Part print with two shaded views. Sizes in mm from the minimum x, y, z corner. A direction names the side the tool comes from. Round coordinates to 2 decimals unless told otherwise and drop trailing zeros. Write each loop counter-clockwise with the first axis right and the second up, starting at its lowest first coordinate (ties: lowest second). Pieces come first, ordered by that corner, then holes.
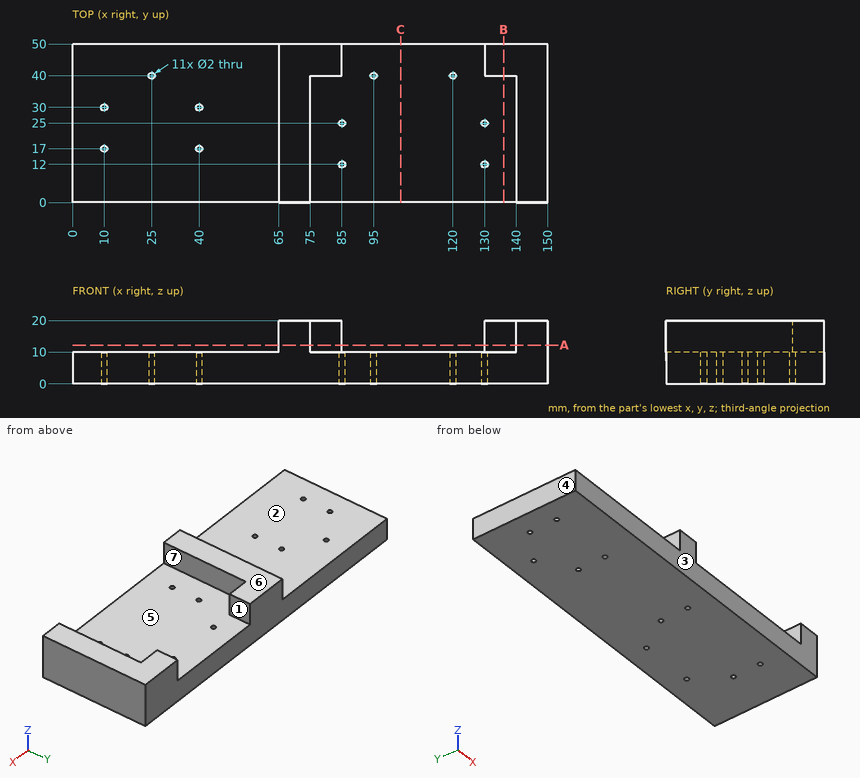
Q1. Wall check: L1, parallel to X at y = 12, z = 5.5; L2, parallel to Y at x = 130, z = 4.25; L3, parallel to Y at x = 10, z = 5.5. Give the ranges that are in metal, low to high.
Values follow:
L1: x = 0 to 84, 86 to 129, 131 to 150
L2: y = 0 to 11, 13 to 24, 26 to 50
L3: y = 0 to 16, 18 to 29, 31 to 50
Q2. Cut at A-A on z = 12.25. Write the cut outline in (x, y), plus the area to 3 significant figures.
Values follow:
outline: (65, 0) - (75, 0) - (75, 40) - (85, 40) - (85, 50) - (65, 50) - close; (130, 40) - (140, 40) - (140, 0) - (150, 0) - (150, 50) - (130, 50) - close
area: 1,200 mm2
Q3. Drop flat-ended pins along their axis: pin 1 (2.5 mm diameter, centred on x = 10, y = 30, fed in from +Z); pin 2 (3 mm diameter, centred on y = 16.5, z = 13.5, fed in from -X). Give the stop position or say it passes through.
Values follow:
pin 1: stops at z = 10
pin 2: stops at x = 65
Q4. Mould opens along X. For the marked faces 4, 5, 6 and 7 say: +X half, -X half, draft (parallel to the pull), parting line (faces both ways), or undercut.
Values follow:
face 4: -X half
face 5: undercut
face 6: draft
face 7: undercut
Q5. Cut at C-C on x = 103.5. Write the cut outline in (y, z), plus the area to 3 significant figures.
Values follow:
outline: (0, 0) - (50, 0) - (50, 10) - (0, 10) - close
area: 500 mm2
Q6. Which spindle directions (+Z, -Z, +X, -X, +Y, -Y) get a long thin tool onto all of the face, cutting with end or side? Do the marked faces 1, 2 and 3. Say none if no direction does.
Values follow:
face 1: +Z, +Y, -Y
face 2: +Z, -X, +Y, -Y
face 3: +Z, -Z, +X, -X, -Y
Q7. Cut at B-B on x = 136. Write the cut outline in (y, z), plus the area to 3 significant figures.
Values follow:
outline: (0, 0) - (50, 0) - (50, 20) - (40, 20) - (40, 10) - (0, 10) - close
area: 600 mm2
